Check sheet for the modelled part. Datum: model origin and axes. Units: mm. A direction names the side the tool comes from. Give positions to 0.01 mm unless a question says otherwise; leave off trailing zeros. Loops run counter-clockwise (first coordinate to the right, second up) from the corner with the lowest first, then second, coordinate; pieces in that order, holes last. Notation, with made-up numbers: (-36, 27.25) -> (2, 27.25) arc R24 cw to (2, 39.25) -> close; hole circle Ø1 at (77, 29.25). An arc over 180 degrees is marked (long way). Answer as CSV lines item,"result". Start each with the question number.
(1) Gauge pin test, flat ends, axial feed: pin 1 Ø3 at (y, z) = (9.5, 1.5) entering from -X; pin 2 Ø1.8 at (y, z) = (3.5, 2.5) entering from +X. Record the tip position at first contact, or that the pin passes through.
(2) Section check D-D on y = 5.5. Enter the section's corners in (x, z), plus the area to 3 significant figures.
(3) Section check C-C on y = 8. Enter the section's corners in (x, z).
(4) Section check B-B on z = 8.25. Enter the section's corners in (x, y), plus the area to 3 significant figures.
(5) Material ranges on line 1 (Y direction, x = 21, z = 7.5); line 2 (Z direction, x = 10, y = 4.5); line 3 (Y direction, x = 15, z = 4.75), recorded low to high. Write a range as from..to.
(6) Access from +Z, -Z, +X, -X, +Y, -Y to the whole of each face (thin tool, end or side, straight path). Record for faces 4 (the face through (19, 6, 4.5)), 5 (the face through (12.8, 6, 5)), 6 (the face through (13.55, 3.04, 7.29)).
(7) Release check for a two-part mould opening along Y. For faces 1 (the face through (19, 10.75, 7)), 2 (the face through (-6, 6, 0)), 3 (the face through (-10.53, 6.08, 4.93)) record: pulls with the +Y half, pulls with the -Y half, needs draft (parallel to the pull), parting line crosses it, or undercut.
(8) Section check A-A on x = 20. Enter the section's corners in (y, z), plus the area to 3 significant figures.
from build123d import *

# Parameters (mm, degrees)
EXTRUDE_1_DEPTH     = 10
SKETCH_2_W          = 24.8
SKETCH_2_H          = 12
EXTRUDE_2_DEPTH     = 4
SKETCH_3_W          = 12
SKETCH_3_H          = 12
EXTRUDE_3_DEPTH     = 1.5
CUT_EXTRUDE_1_DEPTH = 30.309384163


with BuildPart() as part:
    # 草图1 → 凸台-拉伸1 (new body)
    with BuildSketch(Plane.XY):
        Polygon((0, 0), (0, 12), (-10, 12), (-11.070971468, 0), align=None)
    extrude(amount=EXTRUDE_1_DEPTH)

    # 草图2 → 凸台-拉伸2 (add)
    with BuildSketch(Plane.XY.offset(10)):
        with Locations((12.4, 6)):
            Rectangle(SKETCH_2_W, SKETCH_2_H)
    extrude(amount=-EXTRUDE_2_DEPTH)

    # 草图3 → 凸台-拉伸3 (add)
    with BuildSketch(Plane(origin=(0, 0, 6), x_dir=(-1, 0, 0), z_dir=(0, 0, -1))):
        with Locations((-18.8, 6)):
            Rectangle(SKETCH_3_W, SKETCH_3_H)
    extrude(amount=EXTRUDE_3_DEPTH)

    # 草图5 → 切除-拉伸1 (cut, through all)
    with BuildSketch(Plane.XY.offset(10)):
        with BuildLine():
            Line((21.8, 7.25), (15.3, 7.25))
            ThreePointArc((15.3, 7.25), (13.55, 9), (15.3, 10.75))
            Line((15.3, 10.75), (21.8, 10.75))
            ThreePointArc((21.8, 10.75), (23.55, 9), (21.8, 7.25))
        make_face()
        with BuildLine():
            Line((21.8, 4.75), (15.3, 4.75))
            ThreePointArc((15.3, 4.75), (13.55, 3), (15.3, 1.25))
            Line((15.3, 1.25), (21.8, 1.25))
            ThreePointArc((21.8, 1.25), (23.55, 3), (21.8, 4.75))
        make_face()
    extrude(amount=-CUT_EXTRUDE_1_DEPTH, mode=Mode.SUBTRACT)


solid = part.part
Working result:
1,pin 1,"stops at x = -10.36"
1,pin 2,"stops at x = 0"
2,outline,"(-10.58, 0) -> (0, 0) -> (0, 6) -> (12.8, 6) -> (12.8, 4.5) -> (24.8, 4.5) -> (24.8, 10) -> (-10.58, 10) -> close"
2,area,"223 mm^2"
3,outline,"(-10.36, 0) -> (0, 0) -> (0, 6) -> (12.8, 6) -> (12.8, 4.5) -> (13.86, 4.5) -> (13.86, 10) -> (-10.36, 10) -> close; (23.24, 4.5) -> (24.8, 4.5) -> (24.8, 10) -> (23.24, 10) -> close"
4,outline,"(-11.07, 0) -> (24.8, 0) -> (24.8, 12) -> (-10, 12) -> close; hole (15.3, 1.25) -> (21.8, 1.25) arc R1.75 ccw to (21.8, 4.75) -> (15.3, 4.75) arc R1.75 ccw to start; hole (15.3, 7.25) -> (21.8, 7.25) arc R1.75 ccw to (21.8, 10.75) -> (15.3, 10.75) arc R1.75 ccw to start"
4,area,"359 mm^2"
5,line 1,"y = 0..1.25, 4.75..7.25, 10.75..12"
5,line 2,"z = 6..10"
5,line 3,"y = 0..1.28, 4.72..7.28, 10.72..12"
6,face 4,"-Z, +X, +Y, -Y"
6,face 5,"-Z, +Y, -Y"
6,face 6,"+Z, -Z"
7,face 1,"undercut"
7,face 2,"needs draft"
7,face 3,"pulls with the +Y half"
8,outline,"(0, 4.5) -> (1.25, 4.5) -> (1.25, 10) -> (0, 10) -> close; (4.75, 4.5) -> (7.25, 4.5) -> (7.25, 10) -> (4.75, 10) -> close; (10.75, 4.5) -> (12, 4.5) -> (12, 10) -> (10.75, 10) -> close"
8,area,"27.5 mm^2"
